from build123d import *

# Parameters (mm, degrees)
SKETCH_1_W          = 60
SKETCH_1_H          = 70
EXTRUDE_1_DEPTH     = 10
SKETCH_2_R          = 3
CUT_EXTRUDE_1_DEPTH = 48.16990566
CUT_EXTRUDE_START   = -4
SKETCH_3_R          = 7.5
SKETCH_3_R_2        = 3
CUT_EXTRUDE_2_DEPTH = 4
SKETCH_4_R          = 5
CUT_EXTRUDE_3_DEPTH = 1
EXTRUDE_2_DEPTH     = 12.5
SKETCH_7_R          = 9.5
CUT_EXTRUDE_4_DEPTH = 12.5


with BuildPart() as part:
    # 草图1 → 凸台-拉伸1 (new body)
    with BuildSketch(Plane.XY):
        Rectangle(SKETCH_1_W, SKETCH_1_H)
    extrude(amount=EXTRUDE_1_DEPTH)

    # 草图2 → 切除-拉伸1 (cut, through all)
    with BuildSketch(Plane.XY.offset(10)):
        with Locations((-8, 15)):
            Circle(SKETCH_2_R)
        with Locations((7, 15)):
            Circle(SKETCH_2_R)
        with Locations((-8, -15)):
            Circle(SKETCH_2_R)
        with Locations((7, -15)):
            Circle(SKETCH_2_R)
        with Locations((22, 15)):
            Circle(SKETCH_2_R)
        with Locations((22, -15)):
            Circle(SKETCH_2_R)
    extrude(amount=-CUT_EXTRUDE_1_DEPTH, mode=Mode.SUBTRACT)

    # 草图3 → 切除-拉伸2 (cut)
    # profile 1 of 2: a face of its own
    with BuildSketch(Plane(origin=(0, 0, 0), x_dir=(-1, 0, 0), z_dir=(0, 0, -1)).offset(CUT_EXTRUDE_START)):
        with Locations((8, 15)):
            Circle(SKETCH_3_R)
        with Locations(Location((8, 15, 0), (0, 0, 180))):
            Circle(SKETCH_3_R_2, mode=Mode.SUBTRACT)
    # profile 2 of 2: a face of its own
    with BuildSketch(Plane(origin=(0, 0, 0), x_dir=(-1, 0, 0), z_dir=(0, 0, -1)).offset(CUT_EXTRUDE_START)):
        with BuildLine():
            ThreePointArc((8, 7.5), (0.5, 15), (8, 22.5))
            Line((8, 22.5), (-30, 22.5))
            Line((-30, 22.5), (-30, 7.5))
            Line((-30, 7.5), (8, 7.5))
        make_face()
        with Locations(Location((-7, 15, 0), (0, 0, 180))):
            Circle(SKETCH_3_R_2, mode=Mode.SUBTRACT)
    cut_extrude_2 = extrude(amount=CUT_EXTRUDE_2_DEPTH, mode=Mode.SUBTRACT)

    # 镜向1: 切除-拉伸2 across plane
    add(cut_extrude_2.mirror(Plane.ZX), mode=Mode.SUBTRACT)

    # 草图4 → 切除-拉伸3 (cut)
    with BuildSketch(Plane.XY.offset(10)):
        with Locations((-20, 0)):
            Circle(SKETCH_4_R)
        with BuildLine():
            ThreePointArc((-20, -5), (-25, 0), (-20, 5))
            Line((-20, 5), (-30, 5))
            Line((-30, 5), (-30, -5))
            Line((-30, -5), (-20, -5))
        make_face()
    extrude(amount=-CUT_EXTRUDE_3_DEPTH, mode=Mode.SUBTRACT)

    # 草图6 → 凸台-拉伸2 (add)
    with BuildSketch(Plane(origin=(0, 35, 0), x_dir=(1, 0, 0), z_dir=(0, 1, 0))):
        with BuildLine():
            ThreePointArc((30, 0), (20.807611845, 3.807611845), (17, 13))
            ThreePointArc((17, 13), (0, 30), (-17, 13))
            ThreePointArc((-17, 13), (-20.807611845, 3.807611845), (-30, 0))
            Line((-30, 0), (30, 0))
        make_face()
    extrude_2 = extrude(amount=-EXTRUDE_2_DEPTH)

    # 草图7 → 切除-拉伸4 (cut)
    with BuildSketch(Plane(origin=(0, 35, 0), x_dir=(1, 0, 0), z_dir=(0, 1, 0))):
        with Locations((0, 13)):
            Circle(SKETCH_7_R)
        with BuildLine():
            Line((0, 30), (0, 22.5))
            ThreePointArc((0, 22.5), (2.599173089, 22.137521505), (5, 21.077747211))
            Line((5, 21.077747211), (5, 29.248076809))
            ThreePointArc((5, 29.248076809), (2.528111374, 29.810968231), (0, 30))
        make_face()
        with BuildLine():
            ThreePointArc((-5, 21.077747211), (-2.599173089, 22.137521505), (0, 22.5))
            Line((0, 22.5), (0, 30))
            ThreePointArc((0, 30), (-2.528111374, 29.810968231), (-5, 29.248076809))
            Line((-5, 29.248076809), (-5, 21.077747211))
        make_face()
    cut_extrude_4 = extrude(amount=-CUT_EXTRUDE_4_DEPTH, mode=Mode.SUBTRACT)

    # 镜向2: 凸台-拉伸2, 切除-拉伸4 across plane
    add(extrude_2.mirror(Plane.ZX))
    add(cut_extrude_4.mirror(Plane.ZX), mode=Mode.SUBTRACT)


solid = part.part
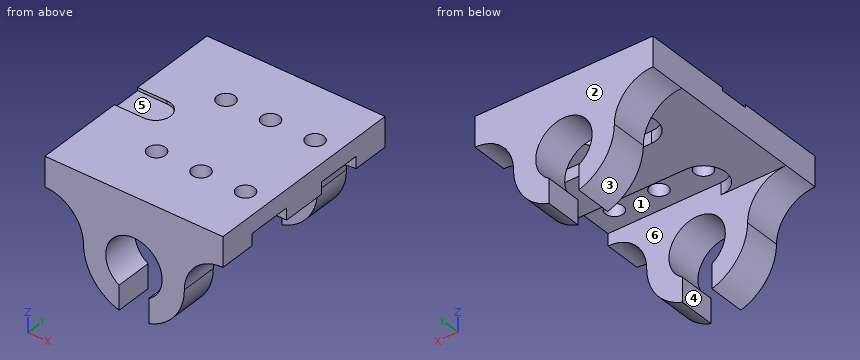
Read the model definition and answer for the solid it produces. Units are mm, in the model's axes. Face numbers are marked on the shaded views. A direction names the side the tool comes from. Give positions to 0.01 mm unless a question says otherwise; leave off trailing zeros. Loops run counter-clockwise (first coordinate to the right, second up) from the corner with the lowest first, then second, coordinate; pieces in that order, holes last. Notation, with made-up numbers: (77, 35.5) -> (133, 35.5) arc R16 cw to (133, 65.5) -> close; hole circle Ø9 at (76.25, 20). An arc over 180 degrees is marked (long way). Answer as CSV lines item,"result".
Item 1: Find section B-B on z = -7. Give the vertices of the cut face in (x, y).
Returned:
outline,"(-18.47, -35) -> (-7.37, -35) -> (-7.37, -22.5) -> (-18.47, -22.5) -> close; (-18.47, 22.5) -> (-7.37, 22.5) -> (-7.37, 35) -> (-18.47, 35) -> close; (7.37, -35) -> (18.47, -35) -> (18.47, -22.5) -> (7.37, -22.5) -> close; (7.37, 22.5) -> (18.47, 22.5) -> (18.47, 35) -> (7.37, 35) -> close"
Item 2: Find section C-C on x = 22. Give the vertices of the cut face in (y, z).
Returned:
outline,"(-35, -2.75) -> (-22.5, -2.75) -> (-22.5, 4) -> (-18, 4) -> (-18, 10) -> (-35, 10) -> close; (-12, 4) -> (-7.5, 4) -> (-7.5, 0) -> (7.5, 0) -> (7.5, 4) -> (12, 4) -> (12, 10) -> (-12, 10) -> close; (18, 4) -> (22.5, 4) -> (22.5, -2.75) -> (35, -2.75) -> (35, 10) -> (18, 10) -> close"
Item 3: Find section D-D on z = 1.5. Give the vertices of the cut face in (x, y).
Returned:
outline,"(-30, -35) -> (30, -35) -> (30, -22.5) -> (-8, -22.5) arc R7.5 cw to (-8, -7.5) -> (30, -7.5) -> (30, 7.5) -> (-8, 7.5) arc R7.5 cw to (-8, 22.5) -> (30, 22.5) -> (30, 35) -> (-30, 35) -> close"
Item 4: Consider line 1 (Y direction, x = 1, z = 3); line 2 (Y direction, x = -8, z = 8.1); line 3 (X direction, y = -25, z = -12.5). Determine where each line is inside the solid, lowest interval first. Write a range as [from, to].
Returned:
line 1,"y = [-35, -22.5], [-7.5, 7.5], [22.5, 35]"
line 2,"y = [-35, -18], [-12, 12], [18, 35]"
line 3,"x = [-17.01, -9.49], [9.49, 17.01]"
Item 5: Determine the mould class of the marked faces 1, 2 and 3 for opening direction Y: +Y half, -Y half, draft (parallel to the pull), parting line (faces both ways), or undercut.
Returned:
face 1,"undercut"
face 2,"+Y half"
face 3,"draft"
Item 6: For the marked faces 4, 5 and 6, determine the directions among +Z, -Z, +X, -X, +Y, -Y from which every point of the face is accessible in a straight line to the end or side of a thin tool.
Returned:
face 4,"-Z, +Y, -Y"
face 5,"+Z, -X"
face 6,"-Z, +X"
Item 7: Find section A-A on y = 15. Give the vertices of the cut face in (x, z).
Returned:
outline,"(-30, 0) -> (-15.5, 0) -> (-15.5, 4) -> (-11, 4) -> (-11, 10) -> (-30, 10) -> close; (-5, 4) -> (4, 4) -> (4, 10) -> (-5, 10) -> close; (10, 4) -> (19, 4) -> (19, 10) -> (10, 10) -> close; (25, 4) -> (30, 4) -> (30, 10) -> (25, 10) -> close"
Item 8: Each of these flat-tipped pins is pushed along its axis until it touches: pin 1 (10 mm diameter, centred on x = -7.5, z = -16, fed in from +Y); pin 2 (1.5 mm diameter, centred on x = -5.5, y = -13.5, fed in from -Z); pin 3 (5 mm diameter, centred on x = -11, y = 4.5, fed in from -Z); pin 4 (4 mm diameter, centred on y = 29.5, z = -26, fed in from -X). Where does it stop, or does it pass through?
Returned:
pin 1,"stops at y = 35"
pin 2,"stops at z = 4"
pin 3,"stops at z = 0"
pin 4,"stops at x = -12.96"
